```python
from build123d import *

# Parameters (mm, degrees)
CROQUIS3_R              = 12.5
SALIENTE_EXTRUIR1_DEPTH = 4
CROQUIS4_R              = 4
SALIENTE_EXTRUIR2_DEPTH = 37
CROQUIS12_OUTSIDE_W     = 37.828
CROQUIS12_OUTSIDE_H     = 37.828
CORTAR_EXTRUIR7_DEPTH   = 25
CROQUIS13_R             = 1.35
CORTAR_EXTRUIR8_DEPTH   = 10
CROQUIS14_R             = 2.5
CORTAR_EXTRUIR9_DEPTH   = 2.2


with BuildPart() as part:
    # Croquis3 → Saliente-Extruir1 (new body)
    with BuildSketch(Plane(origin=(0, 0, 0), x_dir=(1, 0, 0), z_dir=(0, 1, 0))):
        with Locations(Location((0, 0, 0), (0, 0, 270))):
            Circle(CROQUIS3_R)
    extrude(amount=SALIENTE_EXTRUIR1_DEPTH)

    # Croquis4 → Saliente-Extruir2 (add)
    with BuildSketch(Plane(origin=(0, 4, 0), x_dir=(1, 0, 0), z_dir=(0, 1, 0))):
        with Locations(Location((0, 0, 0), (0, 0, 270))):
            Circle(CROQUIS4_R)
    extrude(amount=SALIENTE_EXTRUIR2_DEPTH)

    # Croquis12 outside → Cortar-Extruir7 (cut)
    with BuildSketch(Plane(origin=(0, 41, 0), x_dir=(1, 0, 0), z_dir=(0, 1, 0))):
        Rectangle(CROQUIS12_OUTSIDE_W, CROQUIS12_OUTSIDE_H)
        Polygon((0, 4), (-3.464101615, 2), (-3.464101615, -2), (0, -4), (3.464101615, -2), (3.464101615, 2), align=None, mode=Mode.SUBTRACT)
    extrude(amount=-CORTAR_EXTRUIR7_DEPTH, mode=Mode.SUBTRACT)

    # Croquis13 → Cortar-Extruir8 (cut)
    with BuildSketch(Plane.XZ):
        with Locations(Location((0, 7.875, 0), (0, 0, 270))):
            Circle(CROQUIS13_R)
        with Locations(Location((7.875, 0, 0), (0, 0, 270))):
            Circle(CROQUIS13_R)
        with Locations(Location((0, -7.875, 0), (0, 0, 270))):
            Circle(CROQUIS13_R)
        with Locations(Location((-7.875, 0, 0), (0, 0, 270))):
            Circle(CROQUIS13_R)
    extrude(amount=-CORTAR_EXTRUIR8_DEPTH, mode=Mode.SUBTRACT)

    # Croquis14 → Cortar-Extruir9 (cut)
    with BuildSketch(Plane(origin=(0, 4, 0), x_dir=(1, 0, 0), z_dir=(0, 1, 0))):
        with Locations(Location((0, 7.875, 0), (0, 0, 270))):
            Circle(CROQUIS14_R)
        with Locations(Location((7.875, 0, 0), (0, 0, 270))):
            Circle(CROQUIS14_R)
        with Locations(Location((0, -7.875, 0), (0, 0, 270))):
            Circle(CROQUIS14_R)
        with Locations(Location((-7.875, 0, 0), (0, 0, 270))):
            Circle(CROQUIS14_R)
    extrude(amount=-CORTAR_EXTRUIR9_DEPTH, mode=Mode.SUBTRACT)


solid = part.part
```
The model under review builds one solid part; all positions refer to its coordinate system, in mm. A direction names the side the tool comes from. Round coordinates to 2 decimals unless told otherwise and drop trailing zeros. Write each loop counter-clockwise with the first axis right and the second up, starting at its lowest first coordinate (ties: lowest second). Pieces come first, ordered by that corner, then holes. Notation, with made-up numbers: (-5.5, -1) - (43.5, -1) arc R15 ccw to (43.5, 24) - close; hole circle Ø6 at (-1, 86). An arc over 180 degrees is marked (long way). One line per question, with ' | ' between items.
Item 1: For P1, Ø4.5, axis at x = 0, z = -7.875, coming from the +Y side; P2, Ø12, axis at y = 12, z = 7.5, coming from the -X side; P3, Ø5, axis at x = 3.5, y = 19.5, coming from the +Z side, all flat-tipped, find the tip position at first contact; note any pin that passes through.
Resolved:
P1: stops at y = 1.8 | P2: stops at x = -3.71 | P3: stops at z = 3.42
Item 2: Add section A-A, the plane z = 0. Give the boundary of the cut face in (x, y) (3 decimals), then the cut area to 3 significant figures.
Resolved:
outline: (-12.5, 0) - (-9.225, 0) - (-9.225, 1.8) - (-10.375, 1.8) - (-10.375, 4) - (-12.5, 4) - close; (-6.525, 0) - (6.525, 0) - (6.525, 1.8) - (5.375, 1.8) - (5.375, 4) - (4, 4) - (4, 16) - (3.464, 16) - (3.464, 41) - (-3.464, 41) - (-3.464, 16) - (-4, 16) - (-4, 4) - (-5.375, 4) - (-5.375, 1.8) - (-6.525, 1.8) - close; (9.225, 0) - (12.5, 0) - (12.5, 4) - (10.375, 4) - (10.375, 1.8) - (9.225, 1.8) - close | area: 337 mm2
Item 3: For faces 4 (the face through (-1.1, 1.8, -6.8)), 5 (the face through (1.756, 28.675, -2.986)), 6 (the face through (-1.756, 28.675, 2.986)), 7 (the face through (-1.9, 16, -3.2)), 8 (the face through (1.708, 28.675, 3.014)), list the 3-axis set-ups (+Z, -Z, +X, -X, +Y, -Y) from which the entire face can be reached by the end or side of a thin tool; tool diameter is ignored.
Resolved:
face 4: +Y | face 5: -Z, +X, +Y | face 6: +Z, -X, +Y | face 7: -Z, -X, +Y | face 8: +Z, +X, +Y
Item 4: Add section C-C, the plane z = -8.75. Give the boundary of the cut face in (x, y), then the cut area to 3 significant figures.
Resolved:
outline: (-8.93, 0) - (-1.03, 0) - (-1.03, 1.8) - (-2.34, 1.8) - (-2.34, 4) - (-8.93, 4) - close; (1.03, 0) - (8.93, 0) - (8.93, 4) - (2.34, 4) - (2.34, 1.8) - (1.03, 1.8) - close | area: 57.4 mm2
Item 5: The part is to be moulded in two halves that separate along X. For faces 1 (the face through (-10.316, 2.915, -0.542)), 2 (the face through (1.9, 16, 3.1)), 3 (the face through (-3.905, 9.916, -0.867)), say which applies: pulls with the +X half, pulls with the -X half, needs draft (parallel to the pull), parting line crosses it, or undercut.
Resolved:
face 1: undercut | face 2: needs draft | face 3: parting line crosses it
Item 6: To check wall thickness, follow probe 1 along X at (y, z) = (3, 0) (3 decimals); probe 2 along Y at (x, z) = (7, 8.5); probe 3 along X at (y, z) = (2, -0.5). State the ranges of each line that lie inside material, in increasing order.
Resolved:
probe 1: x = -12.5 to -10.375, -5.375 to 5.375, 10.375 to 12.5 | probe 2: y = 0 to 4 | probe 3: x = -12.49 to -10.32, -5.43 to 5.43, 10.32 to 12.49
Item 7: Add section B-B, the plane y = 27.5. Give the boundary of the cut face in (x, z), then the cut area to 3 significant figures.
Resolved:
outline: (-3.46, -2) - (0, -4) - (3.46, -2) - (3.46, 2) - (0, 4) - (-3.46, 2) - close | area: 41.6 mm2
Item 8: Add section D-D, the plane z = -3. Give the boundary of the cut face in (x, y).
Resolved:
outline: (-12.13, 0) - (12.13, 0) - (12.13, 4) - (2.65, 4) - (2.65, 16) - (1.73, 16) - (1.73, 41) - (-1.73, 41) - (-1.73, 16) - (-2.65, 16) - (-2.65, 4) - (-12.13, 4) - close
